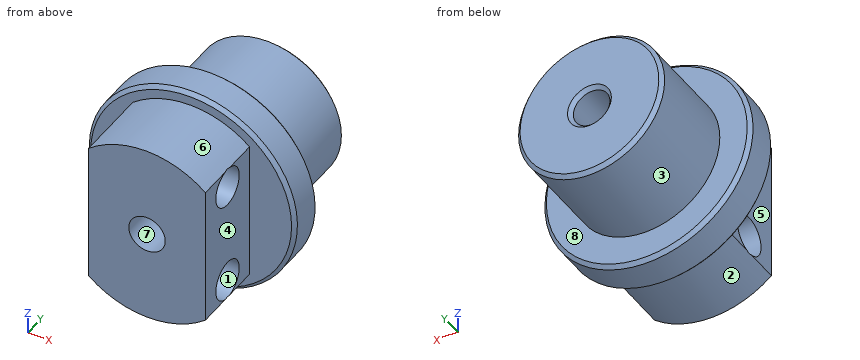
from build123d import *

# Parameters (mm, degrees)
WYTNIJ_WYCI_GNI_CIE1_DEPTH                        = 10
POG_BIENIE_WALCOWE_POD_M5_RUB_Z_BEM_W_D           = 5.3
POG_BIENIE_WALCOWE_POD_M5_RUB_Z_BEM_W_DEPTH       = 60
POG_BIENIE_WALCOWE_POD_M5_RUB_Z_BEM_W_CBORE_D     = 10
POG_BIENIE_WALCOWE_POD_M5_RUB_Z_BEM_W_CBORE_DEPTH = 5
POG_BIENIE_WALCOWE_POD_M5_RUB_Z_BEM_W_TIP         = 1.59228064
OTWORY_USTALAJ_CE_5_0MM1_D                        = 5
SFAZOWANIE1_SIZE                                  = 0.5


with BuildPart() as part:
    # Szkic1 → Obrót1 (revolve)
    with BuildSketch(Plane.XY, mode=Mode.PRIVATE) as obr_t1_sk:
        Polygon((0, 0), (0, 28), (10, 28), (10, 15), (14.25, 15), (14.25, 10), (12.5, 10), (12.5, 0), align=None)
    revolve(obr_t1_sk.sketch.rotate(Axis((0, 0, 0), (0, -1, 0)), 90), axis=Axis((0, 0, 0), (0, -1, 0)))

    # Szkic2 → Wytnij-wyciągnięcie1 (cut)
    with BuildSketch(Plane(origin=(0, 0, 0), x_dir=(-1, 0, 0), z_dir=(0, -1, 0))):
        with BuildLine():
            Line((-8, -9.604686356), (-8, 9.604686356))
            ThreePointArc((-8, 9.604686356), (-12.5, 0), (-8, -9.604686356))
        make_face()
        with BuildLine():
            Line((8, -9.604686356), (8, 9.604686356))
            ThreePointArc((8, 9.604686356), (12.5, 0), (8, -9.604686356))
        make_face()
    extrude(amount=-WYTNIJ_WYCI_GNI_CIE1_DEPTH, mode=Mode.SUBTRACT)

    # Pogłębienie walcowe pod M5 Śrubę z łbem walcowym z gniazdem
    with Locations(Plane(origin=(24.5, 33, -156.349537134), x_dir=(-2.1969032495960934e-12, 0, -1.0), z_dir=(1.0, 0, -2.1969032495960934e-12))):
        with Locations((-163.349537134, -28), (-149.349537134, -28)):
            CounterBoreHole(POG_BIENIE_WALCOWE_POD_M5_RUB_Z_BEM_W_D / 2, POG_BIENIE_WALCOWE_POD_M5_RUB_Z_BEM_W_CBORE_D / 2, POG_BIENIE_WALCOWE_POD_M5_RUB_Z_BEM_W_CBORE_DEPTH, depth=POG_BIENIE_WALCOWE_POD_M5_RUB_Z_BEM_W_DEPTH)
            with Locations((0, 0, -(POG_BIENIE_WALCOWE_POD_M5_RUB_Z_BEM_W_DEPTH + POG_BIENIE_WALCOWE_POD_M5_RUB_Z_BEM_W_TIP / 2))):  # 118° drill point
                Cone(0, POG_BIENIE_WALCOWE_POD_M5_RUB_Z_BEM_W_D / 2, POG_BIENIE_WALCOWE_POD_M5_RUB_Z_BEM_W_TIP, mode=Mode.SUBTRACT)

    # Otwory ustalające Ø5.0mm1 (through all)
    with Locations(Plane(origin=(0, 28, 0), x_dir=(1, 0, 0), z_dir=(0, 1, 0))):
        with Locations((0, 0)):
            Hole(OTWORY_USTALAJ_CE_5_0MM1_D / 2)

    # Sfazowanie1
    sfazowanie1_edges = [part.edges().sort_by_distance(p)[0] for p in [
        (2.5, 28, 0),
        (0, 10, -14.25),
        (0, 15, -14.25),
        (0, 28, -10),
    ]]
    chamfer(sfazowanie1_edges, length=SFAZOWANIE1_SIZE)


solid = part.part
CAD build for the part. Positions are in the model's coordinates, mm. Face numbers are marked on the shaded views. A direction names the side the tool comes from. Coordinates: 2 decimals unless noted, no trailing zeros. Order: outer loops, then holes, each group sorted by start corner. A loop starts at its lowest first (then second) coordinate and runs counter-clockwise, first axis right, second up.
Item 1: Two-plate mould, pull along Z, no slides. Class the marked faces 6, 7 and 8: +Z half, -Z half, draft (parallel to the pull), parting line (faces both ways), or undercut.
Check sheet entries:
face 6: +Z half
face 7: undercut
face 8: draft
Item 2: 3-axis set-ups, long thin cutter, end or side, ignore diameter. For the marked faces 1, 2, 3, 4 and 5: which of +Z, -Z, +X, -X, +Y, -Y reach the whole face in a straight line?
Check sheet entries:
face 1: +X, -X
face 2: -Z, -Y
face 3: +Y
face 4: +Z, -Z, +X, -Y
face 5: +Z, -Z, -X, -Y
Item 3: Band-saw the part on A-A on x = 0. List the corners of the cut face in (y, z), plus the area to 3 significant figures.
Check sheet entries:
outline: (0, -12.5) - (10, -12.5) - (10, -13.75) - (10.5, -14.25) - (14.5, -14.25) - (15, -13.75) - (15, -10) - (27.5, -10) - (28, -9.5) - (28, -3) - (27.5, -2.5) - (0, -2.5) - close; (0, 2.5) - (27.5, 2.5) - (28, 3) - (28, 9.5) - (27.5, 10) - (15, 10) - (15, 13.75) - (14.5, 14.25) - (10.5, 14.25) - (10, 13.75) - (10, 12.5) - (0, 12.5) - close; hole circle Ø5.3 at (5, -7); hole circle Ø5.3 at (5, 7)
area: 467 mm2
Item 4: Band-saw the part on B-B on z = 0. List the corners of the cut face in (x, y).
Check sheet entries:
outline: (-14.25, 10.5) - (-13.75, 10) - (-8, 10) - (-8, 0) - (-2.5, 0) - (-2.5, 27.5) - (-3, 28) - (-9.5, 28) - (-10, 27.5) - (-10, 15) - (-13.75, 15) - (-14.25, 14.5) - close; (2.5, 0) - (8, 0) - (8, 10) - (13.75, 10) - (14.25, 10.5) - (14.25, 14.5) - (13.75, 15) - (10, 15) - (10, 27.5) - (9.5, 28) - (3, 28) - (2.5, 27.5) - close
Item 5: Band-saw the part on C-C on y = 9.25. List the corners of the cut face in (x, z), plus the area to 3 significant figures.
Check sheet entries:
outline: (-8, -9.6) arc R12.5 ccw to (8, -9.6) - (8, 9.6) arc R12.5 ccw to (-8, 9.6) - close; hole circle Ø5 at (0, 0)
area: 351 mm2
Item 6: Band-saw the part on D-D on x = -7. Give the number of separate pieces and of enclosed holes in the cut face, plus the area to 3 significant figures.
Check sheet entries:
separate pieces: 1
enclosed holes: 2
area: 472 mm2
Item 7: Drill centre lines: L1, parallel to Y at x = 3, z = 7; L2, parallel to Z at x = -4.5, y = 5; L3, parallel to Z at x = 1, y = 5. Where is each one in solid material? Low to high.
Check sheet entries:
L1: y = 0 to 2.35, 7.65 to 28
L2: z = -11.66 to -9.65, -4.35 to 4.35, 9.65 to 11.66
L3: z = -12.46 to -9.65, -4.35 to -2.29, 2.29 to 4.35, 9.65 to 12.46
Item 8: Pin check, flat tips, straight feed: pin 1 Ø4 at (y, z) = (5, -7) entering from +X; pin 2 Ø3 at (x, y) = (-2.5, 23) entering from +Z; pin 3 Ø3 at (x, y) = (-4.5, 12.5) entering from -Z; pin 4 Ø8 at (y, z) = (3.5, 3) entering from -X. Stop position of each tip, or through.
Check sheet entries:
pin 1: passes through
pin 2: stops at z = 9.95
pin 3: stops at z = -13.93
pin 4: stops at x = -8
